from build123d import *

# Parameters (mm, degrees)
SKETCH2_R           = 1.6
SKETCH2_R_2         = 1.5
SKETCH2_R_3         = 2.5
BOSS_EXTRUDE1_DEPTH = 4


with BuildPart() as part:
    # Sketch2 → Boss-Extrude1 (new body)
    with BuildSketch(Plane(origin=(0, 0, 0), x_dir=(1, 0, 0), z_dir=(0, 1, 0))):
        with BuildLine():
            Line((-139.142135624, 9.350288425), (-9.350288425, 139.142135624))
            ThreePointArc((-9.350288425, 139.142135624), (-2.861821449, 143.47759065), (4.791847198, 145))
            Line((4.791847198, 145), (97.21825407, 145))
            ThreePointArc((97.21825407, 145), (104.871922717, 143.47759065), (111.360389693, 139.142135624))
            Line((111.360389693, 139.142135624), (139.142135624, 111.360389693))
            ThreePointArc((139.142135624, 111.360389693), (143.47759065, 104.871922717), (145, 97.218254069))
            Line((145, 97.218254069), (145, 4.791847198))
            ThreePointArc((145, 4.791847198), (143.47759065, -2.861821449), (139.142135624, -9.350288426))
            Line((139.142135624, -9.350288426), (9.350288425, -139.142135624))
            ThreePointArc((9.350288425, -139.142135624), (2.861821449, -143.47759065), (-4.791847198, -145))
            Line((-4.791847198, -145), (-85.90454557, -145))
            ThreePointArc((-85.90454557, -145), (-93.558214218, -143.47759065), (-100.046681194, -139.142135624))
            Line((-100.046681194, -139.142135624), (-139.142135624, -100.046681194))
            ThreePointArc((-139.142135624, -100.046681194), (-143.47759065, -93.558214218), (-145, -85.90454557))
            Line((-145, -85.90454557), (-145, -4.791847198))
            ThreePointArc((-145, -4.791847198), (-143.47759065, 2.861821449), (-139.142135624, 9.350288425))
        make_face()
        with Locations((-94.138564286, -64.440079476)):
            Circle(SKETCH2_R, mode=Mode.SUBTRACT)
        with Locations((-64.440079476, -94.138564286)):
            Circle(SKETCH2_R, mode=Mode.SUBTRACT)
        with Locations((-41.272384311, 41.459109088)):
            Circle(SKETCH2_R, mode=Mode.SUBTRACT)
        with Locations((41.459109088, -41.272384311)):
            Circle(SKETCH2_R, mode=Mode.SUBTRACT)
        with Locations((124.190602487, 41.459109088)):
            Circle(SKETCH2_R, mode=Mode.SUBTRACT)
        with Locations((41.459109088, 124.190602487)):
            Circle(SKETCH2_R, mode=Mode.SUBTRACT)
        with Locations((-135.857864376, -58.076118446)):
            Circle(SKETCH2_R, mode=Mode.SUBTRACT)
        with Locations((-58.076118446, -135.857864376)):
            Circle(SKETCH2_R, mode=Mode.SUBTRACT)
        with Locations((-43.226876041, -72.925360851)):
            Circle(SKETCH2_R, mode=Mode.SUBTRACT)
        with Locations((-72.925360851, -43.226876041)):
            Circle(SKETCH2_R, mode=Mode.SUBTRACT)
        with Locations((111.109127035, 111.109127035)):
            Circle(SKETCH2_R_2, mode=Mode.SUBTRACT)
        with Locations((96.966991411, 96.966991411)):
            Circle(SKETCH2_R_2, mode=Mode.SUBTRACT)
        with Locations((-57.015458274, -37.923575182)):
            Circle(SKETCH2_R, mode=Mode.SUBTRACT)
        with Locations((-37.923575182, -57.015458274)):
            Circle(SKETCH2_R, mode=Mode.SUBTRACT)
        with Locations((-18.83169209, -37.923575182)):
            Circle(SKETCH2_R, mode=Mode.SUBTRACT)
        with Locations((-37.923575182, -18.83169209)):
            Circle(SKETCH2_R, mode=Mode.SUBTRACT)
        with Locations((138, 68.86291501)):
            Circle(SKETCH2_R, mode=Mode.SUBTRACT)
        with Locations((118, 68.86291501)):
            Circle(SKETCH2_R, mode=Mode.SUBTRACT)
        with Locations((68.86291501, 138)):
            Circle(SKETCH2_R, mode=Mode.SUBTRACT)
        with Locations((68.86291501, 118)):
            Circle(SKETCH2_R, mode=Mode.SUBTRACT)
        with Locations((-9.099025767, 125.251262658)):
            Circle(SKETCH2_R, mode=Mode.SUBTRACT)
        with Locations((125.251262658, -9.099025767)):
            Circle(SKETCH2_R, mode=Mode.SUBTRACT)
        with Locations((77.521554928, 23.074332777)):
            Circle(SKETCH2_R_3, mode=Mode.SUBTRACT)
        with Locations((71.864700679, 17.417478528)):
            Circle(SKETCH2_R_3, mode=Mode.SUBTRACT)
        with Locations((43.933982822, 135.857864376)):
            Circle(SKETCH2_R, mode=Mode.SUBTRACT)
        with Locations((135.857864376, 43.933982822)):
            Circle(SKETCH2_R, mode=Mode.SUBTRACT)
        with Locations((18.124585309, 34.388041276)):
            Circle(SKETCH2_R_3, mode=Mode.SUBTRACT)
        with Locations((46.408856556, 62.672312523)):
            Circle(SKETCH2_R_3, mode=Mode.SUBTRACT)
        with Locations((-95.435846132, 31.843374482)):
            Circle(SKETCH2_R_3, mode=Mode.SUBTRACT)
        with Locations((-84.829244414, 21.236772764)):
            Circle(SKETCH2_R_3, mode=Mode.SUBTRACT)
        with Locations((85, 68.86291501)):
            Circle(SKETCH2_R_3, mode=Mode.SUBTRACT)
        with Locations((100, 68.86291501)):
            Circle(SKETCH2_R_3, mode=Mode.SUBTRACT)
        with Locations((37.570021791, -58.59650045)):
            Circle(SKETCH2_R_3, mode=Mode.SUBTRACT)
        with Locations((7.684812205, -84.23906935)):
            Circle(SKETCH2_R_3, mode=Mode.SUBTRACT)
        with Locations((0.613744393, -91.310137162)):
            Circle(SKETCH2_R_3, mode=Mode.SUBTRACT)
        with BuildLine():
            Line((-19.18524548, 16.170093579), (16.170093579, -19.18524548))
            ThreePointArc((16.170093579, -19.18524548), (16.170093579, -40.398448916), (-5.043109857, -40.398448916))
            Line((-5.043109857, -40.398448916), (-40.398448916, -5.043109857))
            ThreePointArc((-40.398448916, -5.043109857), (-40.398448916, 16.170093579), (-19.18524548, 16.170093579))
        make_face(mode=Mode.SUBTRACT)
    extrude(amount=BOSS_EXTRUDE1_DEPTH)


solid = part.part
Geometry check sheet. Reference: the model listing, model coordinates, mm. A direction names the side the tool comes from. Give positions to 0.01 mm unless a question says otherwise; leave off trailing zeros. Order: outer loops, then holes, each group sorted by start corner. A loop starts at its lowest first (then second) coordinate and runs counter-clockwise, first axis right, second up.
1. Access from +Z, -Z, +X, -X, +Y, -Y to the whole of each face (thin tool, end or side, straight path). Record for faces 4 (the face through (2, 4, -2)), 5 (the face through (-1.755, 1.972, 1.26)).
Completed:
face 4: +Z, -Z, +X, -X, +Y
face 5: +Y, -Y
2. Depth check by flat-ended pin: pin 1 (1 mm diameter, centred on x = 23.5, z = 73.5, fed in from -Y); pin 2 (1 mm diameter, centred on x = 41, y = 2, fed in from +Z). Enter the tip coordinate at first touch or a pass-through.
Completed:
pin 1: stops at y = 0
pin 2: stops at z = 107.99
3. Draft check along X on faces 1 (the face through (125.1, 2, -125.4)), 2 (the face through (-40.629, 1.972, -15.934)), 3 (the face through (-75.15, 1.97, -73.34)). Enter one of: pulls with the +X half, pulls with the -X half, needs draft (parallel to the pull), parting line crosses it, or undercut.
Completed:
face 1: pulls with the +X half
face 2: undercut
face 3: pulls with the -X half
4. Scan lines: line 1 (X direction, y = 2.5, z = 42); line 2 (X direction, y = 2.65, z = -23.5); line 3 (Z direction, x = -43, y = 3.7). Record each from-to range of solid material in increasing order.
Completed:
line 1: x = -145 to -73.95, -71.9 to -3.15, 14.28 to 40.03, 42.88 to 106.49
line 2: x = -124.99 to -85.89, -83.77 to 75.06, 79.99 to 145
line 3: z = -105.49 to -12.67, 1.55 to 71.34, 74.51 to 145
5. Sectioned sample at A-A (y = 0.9). State how many separate pieces and enclosed holes the cut face has, then the cut area to 3 significant figures.
Completed:
separate pieces: 1
enclosed holes: 36
area: 59,300 mm2
6. Sectioned sample at B-B (z = -53.5). Record the boundary of the cut face in (x, y).
Completed:
outline: (-94.99, 0) - (145, 0) - (145, 4) - (-94.99, 4) - close
